```python
from build123d import *

# Parameters (mm, degrees)
F0_R           = 2.413
F1_DEPTH       = 6.35
F3_D           = 3.175
F3_DEPTH       = 15.875
F3_CBORE_D     = 5.334
F3_CBORE_DEPTH = 6.35
F3_TIP         = 0.9538662327
F5_D           = 3.175
F5_DEPTH       = 15.875
F5_CBORE_D     = 5.334
F5_CBORE_DEPTH = 6.35
F5_TIP         = 0.9538662327


# Not quite as in the source:
# - ends of sketch curves that miss each other by under 0.0002 mm in the source are joined


with BuildPart() as f1:
    # F0 (on Top) → F1 (new body)
    with BuildSketch(Plane.XY):
        with BuildLine():
            Line((69.85, 50.8), (-69.85, 50.8))
            ThreePointArc((-69.85, 50.8), (-74.3401280605, 48.9401280605), (-76.2, 44.45))
            Line((-76.2, 44.45), (-76.2, -44.45))
            ThreePointArc((-76.2, -44.45), (-74.3401280605, -48.9401280605), (-69.85, -50.8))
            Line((-69.85, -50.8), (69.85, -50.8))
            ThreePointArc((69.85, -50.8), (74.3401280605, -48.9401280605), (76.2, -44.45))
            Line((76.2, -44.45), (76.2, -14.2860641539))
            ThreePointArc((76.2, -14.2860641539), (74.3401280605, -9.7959360934), (69.85, -7.9360641539))
            Line((69.85, -7.9360641539), (58.6074946763, -7.9360641539))
            ThreePointArc((58.6074946763, -7.9360641539), (54.1173666157, -9.7959360934), (52.2574946763, -14.2860641539))
            Line((52.2574946763, -14.2860641539), (52.2574946763, -32.4625809134))
            ThreePointArc((52.2574946763, -32.4625809134), (50.8625907217, -35.8301769588), (47.4949946763, -37.2250809134))
            Line((47.4949946763, -37.2250809134), (44.3277485112, -37.2250809134))
            ThreePointArc((44.3277485112, -37.2250809134), (42.13331562, -36.5581056788), (40.5040542932, -34.9438258992))
            Line((40.5040542932, -34.9438258992), (33.1534721252, -34.9569741008))
            ThreePointArc((33.1534721252, -34.9569741008), (31.4174339307, -36.6267371458), (29.0867928871, -37.2350541396))
            Line((29.0867928871, -37.2350541396), (-32.0008653101, -37.2349356495))
            ThreePointArc((-32.0008653101, -37.2349356495), (-32.011823158, -37.2349229987), (-32.0227809478, -37.23488518))
            ThreePointArc((-32.0227809478, -37.23488518), (-34.343480333, -36.6189475252), (-36.0687477759, -34.9490741523))
            Line((-36.0687477759, -34.9490741523), (-43.4277583378, -34.9532397009))
            ThreePointArc((-43.4277583378, -34.9532397009), (-48.8402121166, -37.0437819519), (-52.2557695883, -32.3534738631))
            Line((-52.2557695883, -32.3534738631), (-52.2557695883, 32.3534738631))
            ThreePointArc((-52.2557695883, 32.3534738631), (-48.8402121166, 37.0437819519), (-43.4277583378, 34.9532397009))
            Line((-43.4277583378, 34.9532397009), (-36.0798295377, 34.9490804251))
            ThreePointArc((-36.0798295377, 34.9490804251), (-34.3499401325, 36.6220397206), (-32.0227811798, 37.2349356069))
            Line((-32.0227811798, 37.2349356069), (29.0868021404, 37.2350541396))
            ThreePointArc((29.0868021404, 37.2350541396), (31.4174339307, 36.6267371458), (33.1534721252, 34.9569741008))
            Line((33.1534721252, 34.9569741008), (40.5040542932, 34.9438258992))
            ThreePointArc((40.5040542932, 34.9438258992), (42.13331562, 36.5581056788), (44.3277485112, 37.2250809134))
            Line((44.3277485112, 37.2250809134), (47.4949946763, 37.2250809134))
            ThreePointArc((47.4949946763, 37.2250809134), (50.8625907217, 35.8301769588), (52.2574946763, 32.4625809134))
            Line((52.2574946763, 32.4625809134), (52.2574946763, 23.8139358461))
            ThreePointArc((52.2574946763, 23.8139358461), (54.1173666157, 19.3238077856), (58.6074946763, 17.4639358461))
            Line((58.6074946763, 17.4639358461), (69.85, 17.4639358461))
            ThreePointArc((69.85, 17.4639358461), (74.3401280605, 19.3238077856), (76.2, 23.8139358461))
            Line((76.2, 23.8139358461), (76.2, 44.45))
            ThreePointArc((76.2, 44.45), (74.3401280605, 48.9401280605), (69.85, 50.8))
        make_face()
        with Locations((-69.85, -44.45)):
            Circle(F0_R, mode=Mode.SUBTRACT)
        with Locations((69.85, -44.45)):
            Circle(F0_R, mode=Mode.SUBTRACT)
        with Locations((69.85, -14.2860641539)):
            Circle(F0_R, mode=Mode.SUBTRACT)
        with Locations((-69.85, 44.45)):
            Circle(F0_R, mode=Mode.SUBTRACT)
        with Locations((69.85, 23.8139358461)):
            Circle(F0_R, mode=Mode.SUBTRACT)
        with Locations((69.85, 44.45)):
            Circle(F0_R, mode=Mode.SUBTRACT)
    extrude(amount=F1_DEPTH)

    # F3
    with Locations(Plane.XZ.offset(50.8)):
        with Locations((-39.9796, 3.175), (36.6377, 3.175)):
            CounterBoreHole(F3_D / 2, F3_CBORE_D / 2, F3_CBORE_DEPTH, depth=F3_DEPTH)
            with Locations((0, 0, -(F3_DEPTH + F3_TIP / 2))):  # 118° drill point
                Cone(0, F3_D / 2, F3_TIP, mode=Mode.SUBTRACT)

    # F5
    with Locations(Plane(origin=(0, 50.8, 0), x_dir=(-1, 0, 0), z_dir=(0, 1, 0))):
        with Locations((-36.6268, 3.175), (39.9796, 3.175)):
            CounterBoreHole(F5_D / 2, F5_CBORE_D / 2, F5_CBORE_DEPTH, depth=F5_DEPTH)
            with Locations((0, 0, -(F5_DEPTH + F5_TIP / 2))):  # 118° drill point
                Cone(0, F5_D / 2, F5_TIP, mode=Mode.SUBTRACT)


solid = f1.part
```
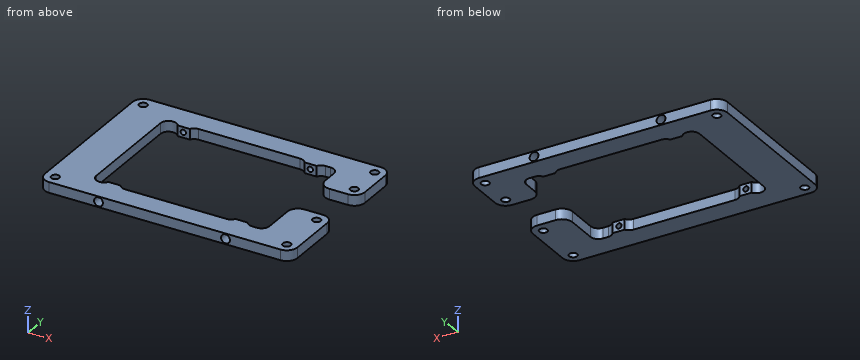
The listing builds one solid part. Answer for the finished solid, in the listing's coordinates (mm). Coordinates: 2 decimals unless noted, no trailing zeros. Loops run counter-clockwise (first coordinate to the right, second up) from the corner with the lowest first, then second, coordinate; pieces in that order, holes last. Notation, with made-up numbers: M 77.25,-12.5 L 129.25,-12.5 A16 ccw 129.25,5.5 Z; hole C 13.5,61.5 d9. An arc over 180 degrees is marked long. Answer as a JSON object with one key per item and string values. Group by question number.
Item 1: Consider L1, parallel to Y at x = -69.85, z = 2; L2, parallel to Y at x = 70, z = 1.25; L3, parallel to Y at x = 62, z = 2. Determine where each line is inside the solid, lowest interval first.
Item 2: Section A-A (y = 4.5) is taken. Write down the section's boundary in (x, z), and give its area (3 significant figures).
Item 3: Each of these flat-tipped pins is pushed along its axis until it touches: P1, Ø3, axis at x = -69.85, y = -44.45, coming from the +Z side; P2, Ø3, axis at y = 10, z = 4.5, coming from the +X side; P3, Ø3, axis at y = -8.5, z = 3.5, coming from the +X side. Where does it stop, or does it pass through?
Solved:
{
 "1": {"L1": "y = -50.8 to -46.86, -42.04 to 42.04, 46.86 to 50.8", "L2": "y = -50.8 to -46.86, -42.04 to -16.69, -11.88 to -7.94, 17.47 to 21.41, 26.22 to 42.04, 46.86 to 50.8", "L3": "y = -50.8 to -7.94, 17.46 to 50.8"},
 "2": {"outline": "M -76.2,0 L -52.26,0 L -52.26,6.35 L -76.2,6.35 Z", "area": "152 mm2"},
 "3": {"P1": "passes through", "P2": "stops at x = -52.26", "P3": "stops at x = 74.54"}
}
